Check sheet for the modelled part. Datum: model origin and axes. Units: mm. A direction names the side the tool comes from. Round coordinates to 2 decimals unless told otherwise and drop trailing zeros. Write each loop counter-clockwise with the first axis right and the second up, starting at its lowest first coordinate (ties: lowest second). Pieces come first, ordered by that corner, then holes. Notation, with made-up numbers: M 18.25,2.5 L 31.25,2.5 A27 ccw 31.25,24.5 Z; hole C 54.5,-25 d10. An arc over 180 degrees is marked long. One line per item, written item: value.
from build123d import *

# Parameters (mm, degrees)
ESQUISSE3_R                         = 3
BOSS_EXTRU_1_DEPTH                  = 20.25
ENL_V_MAT_EXTRU_2_DEPTH             = 55.83668936
ENL_V_MAT_EXTRU_2_DEPTH_BACK        = 55.83668936
ESQUISSE5_W                         = 24.5
ESQUISSE5_H                         = 30.5
ENL_V_MAT_EXTRU_3_DEPTH             = 66.094162565
ENL_V_MAT_EXTRU_3_DEPTH_BACK        = 66.094162565
ENL_V_MAT_EXTRU_6_DEPTH             = 66.094162565
TROU_TARAUD_M2_51_D                 = 2.05
TROU_TARAUD_M2_51_DEPTH             = 5
DIAM_TRE_DU_PER_AGE_2_1_2_1_1_D     = 2.1
DIAM_TRE_DU_PER_AGE_2_1_2_1_1_DEPTH = 1.8
DIAM_TRE_DU_PER_AGE_2_1_2_1_1_TIP   = 0.63090365
ESQUISSE16_R                        = 1.025
ENL_V_MAT_EXTRU_7_DEPTH             = 52.293883791
ENL_V_START                         = -15
ESQUISSE17_R                        = 2
ENL_V_MAT_EXTRU_9_DEPTH             = 10
CONG_1_R                            = 1


with BuildPart() as part:
    # Esquisse3 → Boss.-Extru.1 (new, symmetric)
    with BuildSketch(Plane(origin=(0, 0, 0), x_dir=(1, 0, 0), z_dir=(0, 1, 0))):
        with BuildLine():
            Line((-14, 0), (-14, -35))
            ThreePointArc((-14, -35), (0, -49), (14, -35))
            Line((14, -35), (14, 0))
            Line((14, 0), (-14, 0))
        make_face()
        with Locations(Location((0, -35, 0), (0, 0, 270))):
            Circle(ESQUISSE3_R, mode=Mode.SUBTRACT)
    extrude(amount=BOSS_EXTRU_1_DEPTH, both=True)

    # Esquisse5 → Enlèv. mat.-Extru.2 (cut, two sides: drawn at the far end of the back side and taken through both)
    with BuildSketch(Plane(origin=(0, 0, 0), x_dir=(0, 0, -1), z_dir=(1, 0, 0)).offset(-ENL_V_MAT_EXTRU_2_DEPTH_BACK)):
        with Locations((-36.75, 0)):
            Rectangle(ESQUISSE5_W, ESQUISSE5_H)
    extrude(amount=ENL_V_MAT_EXTRU_2_DEPTH + ENL_V_MAT_EXTRU_2_DEPTH_BACK, mode=Mode.SUBTRACT)

    # Esquisse6 → Enlèv. mat.-Extru.3 (cut, two sides: drawn at the far end of the back side and taken through both)
    with BuildSketch(Plane(origin=(0, -20.25, 0), x_dir=(1, 0, 0), z_dir=(0, 1, 0)).offset(-ENL_V_MAT_EXTRU_3_DEPTH_BACK)):
        Polygon((-8.7, 0), (-8.7, -7.479156707), (-5.5, -7.479156707), (-5.5, -18.5), (5.5, -18.5), (5.5, -7.221861732), (8.7, -7.221861732), (8.7, 0), align=None)
    extrude(amount=ENL_V_MAT_EXTRU_3_DEPTH + ENL_V_MAT_EXTRU_3_DEPTH_BACK, mode=Mode.SUBTRACT)

    # Esquisse11 → Enlèv. mat.-Extru.6 (cut, through all)
    with BuildSketch(Plane.XZ.offset(20.25)):
        with BuildLine():
            Line((14, 14.792740578), (14, 35))
            ThreePointArc((14, 35), (0, 49), (-14, 35))
            Line((-14, 35), (-14, 14.792740578))
            ThreePointArc((-14, 14.792740578), (-12.968272988, 17.999691858), (-10.260168543, 20.003480132))
            ThreePointArc((-10.260168543, 20.003480132), (-6.735867006, 23.689629257), (-7.755056184, 28.686593346))
            ThreePointArc((-7.755056184, 28.686593346), (0, 45), (7.755056184, 28.686593346))
            ThreePointArc((7.755056184, 28.686593346), (6.735867006, 23.689629257), (10.260168543, 20.003480132))
            ThreePointArc((10.260168543, 20.003480132), (12.968272988, 17.999691858), (14, 14.792740578))
        make_face()
    extrude(amount=-ENL_V_MAT_EXTRU_6_DEPTH, mode=Mode.SUBTRACT)

    # Trou taraudé M2.51
    with Locations(Plane.XZ.offset(20.25)):
        with Locations((0, 28.5), (-5.629165125, 38.25), (5.629165125, 38.25)):
            Hole(TROU_TARAUD_M2_51_D / 2, depth=TROU_TARAUD_M2_51_DEPTH)

    # Diamètre du perçage Ø2.1 (2.1)1
    with Locations(Plane.XY.offset(45)):
        with Locations((0, 17.75)):
            Hole(DIAM_TRE_DU_PER_AGE_2_1_2_1_1_D / 2, depth=DIAM_TRE_DU_PER_AGE_2_1_2_1_1_DEPTH)
            with Locations((0, 0, -(DIAM_TRE_DU_PER_AGE_2_1_2_1_1_DEPTH + DIAM_TRE_DU_PER_AGE_2_1_2_1_1_TIP / 2))):  # 118° drill point
                Cone(0, DIAM_TRE_DU_PER_AGE_2_1_2_1_1_D / 2, DIAM_TRE_DU_PER_AGE_2_1_2_1_1_TIP, mode=Mode.SUBTRACT)

    # Esquisse16 → Enlèv. mat.-Extru.7 (cut, through all)
    with BuildSketch(Plane(origin=(0, 0, 0), x_dir=(-1, 0, 0), z_dir=(0, 0, -1))):
        with Locations((-11.5, 8.7)):
            Circle(ESQUISSE16_R)
        with Locations((11.5, 8.7)):
            Circle(ESQUISSE16_R)
        with Locations((-11.5, -8.7)):
            Circle(ESQUISSE16_R)
        with Locations((11.5, -8.7)):
            Circle(ESQUISSE16_R)
    extrude(amount=-ENL_V_MAT_EXTRU_7_DEPTH, mode=Mode.SUBTRACT)

    # Esquisse17 → Enlèv. mat.-Extru.9 (cut)
    with BuildSketch(Plane(origin=(0, 0, 0), x_dir=(-1, 0, 0), z_dir=(0, 0, -1)).offset(ENL_V_START)):
        with Locations((11.5, 8.7)):
            Circle(ESQUISSE17_R)
        with Locations((11.5, -8.7)):
            Circle(ESQUISSE17_R)
        with Locations((-11.5, -8.7)):
            Circle(ESQUISSE17_R)
        with Locations((-11.5, 8.7)):
            Circle(ESQUISSE17_R)
    extrude(amount=-ENL_V_MAT_EXTRU_9_DEPTH, mode=Mode.SUBTRACT)

    # Congé1
    cong_1_edges = [part.edges().sort_by_distance(p)[0] for p in [
        (5.5, 0, 7.221861732),
        (5.5, 0, 18.5),
        (-5.5, 0, 18.5),
        (-5.5, 0, 7.479156707),
        (8.7, 0, 7.221861732),
        (-8.7, 0, 7.479156707),
        (0, 15.25, 24.5),
        (0, -15.25, 24.5),
    ]]
    fillet(cong_1_edges, radius=CONG_1_R)


solid = part.part
Q1. Depth check by flat-ended pin: P1, Ø4.5, axis at x = -11, y = -9.5, coming from the +Z side; P2, Ø4, axis at x = 7, y = -13.5, coming from the -Z side; P3, Ø10.5, axis at x = -2.5, y = 3, coming from the +Z side; P4, Ø1, axis at x = 6.5, y = 1, coming from the -Z side. Enter the tip coordinate at first touch or a pass-through.
Completed:
P1: z = 20.79
P2: z = 0
P3: z = 24.5
P4: z = 7.22
Q2. Sectioned sample at D-D on y = 3.5. Enter the section's corners in (x, z).
Completed:
outline: M -14,0 L -8.7,0 L -8.7,6.48 A1 cw -7.7,7.48 L -6.5,7.48 A1 ccw -5.5,8.48 L -5.5,17.5 A1 cw -4.5,18.5 L 4.5,18.5 A1 cw 5.5,17.5 L 5.5,8.22 A1 ccw 6.5,7.22 L 7.7,7.22 A1 cw 8.7,6.22 L 8.7,0 L 14,0 L 14,14.79 A5.5 ccw 10.26,20 A5.5 cw 6.57,24.5 L -6.57,24.5 A5.5 cw -10.26,20 A5.5 ccw -14,14.79 Z
Q3. Sectioned sample at A-A on z = 11. Enter the section's corners in (x, y) (3 decimals).
Completed:
outline: M -14,-20.25 L -5.5,-20.25 L -5.5,20.25 L -14,20.25 Z; M 5.5,-20.25 L 14,-20.25 L 14,20.25 L 5.5,20.25 Z; hole C -11.5,-8.7 d2.05; hole C -11.5,8.7 d2.05; hole C 11.5,-8.7 d2.05; hole C 11.5,8.7 d2.05
Q4. Sectioned sample at B-B on x = 11.5. Enter the section's corners in (y, z) (3 decimals), and give its area (3 significant figures).
Completed:
outline: M -20.25,0 L -9.725,0 L -9.725,15 L -10.7,15 L -10.7,19.403 L -20.25,19.403 Z; M -7.675,0 L 7.675,0 L 7.675,15 L 6.7,15 L 6.7,19.403 L -6.7,19.403 L -6.7,15 L -7.675,15 Z; M 9.725,0 L 20.25,0 L 20.25,19.403 L 10.7,19.403 L 10.7,15 L 9.725,15 Z
area: 689 mm^2
Q5. Sectioned sample at C-C on z = 35. Enter the section's corners in (x, y), and give its area (3 significant figures).
Completed:
outline: M -10,-20.25 L -3,-20.25 L -3,-15.25 L -10,-15.25 Z; M -10,15.25 L -3,15.25 L -3,20.25 L -10,20.25 Z; M 3,-20.25 L 10,-20.25 L 10,-15.25 L 3,-15.25 Z; M 3,15.25 L 10,15.25 L 10,20.25 L 3,20.25 Z
area: 140 mm^2
Q6. Draft check along Y on faces 6 (the cylindrical face through (0.133, -17.715, 29.516)), 7 (the flat face through (0, 20.25, 22)), 8 (the flat face through (-11, 10, 15)). Enter one of: pulls with the +Y half, pulls with the -Y half, needs draft (parallel to the pull), parting line crosses it, or undercut.
Completed:
face 6: needs draft
face 7: pulls with the +Y half
face 8: undercut
Q7. Access from +Z, -Z, +X, -X, +Y, -Y to the whole of each face (thin tool, end or side, straight path). Record for faces 1 (the cylindrical face through (-10.74, -8.01, 7.4)), 2 (the flat face through (-5.5, 0, 13)), 3 (the cylindrical face through (-5.496, -17.715, 39.266)), 4 (the cylindrical face through (-9.502, 8.788, 17.034)), 5 (the flat face through (0, 0, 24.5)).
Completed:
face 1: +Z, -Z
face 2: -Z, +Y, -Y
face 3: -Y
face 4: +Z
face 5: +Z, +X, -X
Q8. Scan lines: line 1 (Y direction, x = -11.5, z = 5.25) (3 decimals); line 2 (Y direction, x = -11.5, z = 16.65); line 3 (Y direction, x = -0.75, z = 27.5). Record each from-to range of solid material in increasing order. Write a range as [from, to].
Completed:
line 1: [-20.25, -9.725], [-7.675, 7.675], [9.725, 20.25]
line 2: [-20.25, -10.7], [-6.7, 6.7], [10.7, 20.25]
line 3: [-20.25, -15.25], [15.25, 20.25]
